Model file for the job. Use its own axes, mm. Face numbers are marked on the shaded views. A direction names the side the tool comes from. Coordinates: 2 decimals unless noted, no trailing zeros. Write each loop counter-clockwise with the first axis right and the second up, starting at its lowest first coordinate (ties: lowest second). Pieces come first, ordered by that corner, then holes. Notation, with made-up numbers: M -26.5,0 L 31.5,0 A3 ccw 31.5,5 Z; hole C 60.5,54 d5. An arc over 180 degrees is marked long. Put each result on its own line as item: value. Start each with the question number.
Q1. Drop flat-ended pins along their axis: pin 1 (5 mm diameter, centred on y = 238.5, z = 1.5, fed in from -X); pin 2 (6.5 mm diameter, centred on y = 335, z = 1.5, fed in from -X); pin 3 (5.5 mm diameter, centred on x = -24.5, y = 272, fed in from -Z); pin 4 (7 mm diameter, centred on y = 260, z = 141, fed in from -X). Give the stop position or say it passes through.
Q2. Which spindle directions (+Z, -Z, +X, -X, +Y, -Y) get a long thin tool onto all of the face, cutting with end or side? Do the marked faces 1 and 2. Say none if no direction does.
Q3. Cut at D-D (y = 188). Write the cut outline in (x, z).
Q4. Drill centre lines: line 1 along Y through (x, z) = (-2, 108); line 2 along Z through (x, y) = (-15, 181); line 3 along X through (y, z) = (195, 145.5). Where is each one in solid material? Low to high.
Q5. Cut at C-C (z = 108.38). Write the cut outline in (x, y), then the cut area to 3 significant figures.
Q6. Cut at A-A (z = 141). Write the cut outline in (x, y).
Q7. Cut at B-B (y = 230). Write the cut outline in (x, z).
Autodesk Inventor part; units mm, degrees
ref_plane "Work Plane1" through (-6, 230, 6) normal (0, -1, 0) x (1, 0, 0)
ref_plane "Work Plane2" through (-6, 190, 6) normal (0, -1, 0) x (1, 0, 0)
ref_plane "YZ Plane" through (0, 0, 0) normal (1, 0, 0) x (0, 1, 0)
sketch "Sketch1" plane through (0, 0, 0) normal (0, 0, 1) x (1, 0, 0)
  line L0 (0, 343) -> (-48.5, 343)
  line L1 (0, 343) -> (0, 113)
  line L2 (0, 113) -> (-48.5, 113)
  line L3 (-48.5, 113) -> (-48.5, 148)
  line L4 (-48.5, 148) -> (-32.5, 148)
  line L5 (-32.5, 148) -> (-32.5, 203)
  line L6 (-32.5, 203) -> (-13, 203)
  line L7 (-13, 203) -> (-13, 258)
  line L8 (-13, 258) -> (-32.5, 258)
  line L9 (-32.5, 258) -> (-32.5, 313)
  line L10 (-32.5, 313) -> (-48.5, 313)
  line L11 (-48.5, 313) -> (-48.5, 343)
  point P0 (0, 0)
  dimension "d0" = 230
  dimension "d1" = 13
  dimension "d2" = 30
  dimension "d3" = 55
  dimension "d4" = 55
  dimension "d5" = 55
  dimension "d6" = 16
extrude "Extrusion1" add sketch "Sketch1" along normal blind 6
fillet "Fillet1" radius 7 8 edges at (-32.5, 148, 3) (-32.5, 203, 3) (-13, 203, 3) (-13, 258, 3) (-32.5, 258, 3) (-32.5, 313, 3) (-48.5, 313, 3) (-48.5, 148, 3)
sketch "Sketch2" plane through (0, 0, 6) normal (0, 0, 1) x (1, 0, 0)
  line L0 (0, 113) -> (0, 343)
  line L1 (-6, 180) -> (0, 180)
  line L2 (0, 180) -> (0, 280)
  line L3 (0, 280) -> (-6, 280)
  line L4 (-6, 280) -> (-6, 180)
  line L5 (-15.5, 205) -> (-48.5, 205) construction
  line L6 (-48.5, 255) -> (-15.5, 255) construction
  line L7 (-15.5, 255) -> (-15.5, 205) construction
  line L8 (-15.5, 230) -> (0, 230) construction
  point P0 (0, 0)
  dimension "d10" = 100
  dimension "d11" = 6
extrude "Extrusion2" add sketch "Sketch2" along normal blind 241
sketch "Sketch3" plane through (-6, 180, 6) normal (-1, 0, 0) x (0, 0, 1)
  line L0 (241, 0) -> (241, 100)
  line L1 (235, 0) -> (235, 100)
  line L2 (241, 100) -> (241, 0)
  line L3 (241, 100) -> (241, 0)
  line L4 (241, 0) -> (241, -10)
  line L5 (241, -10) -> (235, -10)
  line L6 (235, -10) -> (235, 0)
  line L7 (235, 100) -> (235, 110)
  line L8 (235, 110) -> (241, 110)
  line L9 (0, 100) -> (241, 100) construction
  line L10 (241, 110) -> (241, 100)
  point P0 (-6, -180)
  dimension "d14" = 6
  dimension "d17" = 10
  dimension "d18" = 10
extrude "Extrusion3" add sketch "Sketch3" along normal blind 85
sketch "Sketch4" plane through (0, 0, 247) normal (0, 0, 1) x (1, 0, 0)
  line L0 (-37.6569, 174.8457) -> (-87.1543, 224.3431) construction
  line L1 (-87.1543, 235.6569) -> (-37.6569, 285.1543) construction
  line L2 (-40.4853, 172.0172) -> (-89.9828, 221.5147)
  line L3 (-91, 237.468) -> (-40.4853, 287.9828)
  line L4 (-89.9828, 221.5147) -> (-91, 222.532)
  line L5 (-91, 170) -> (-91, 290)
  line L6 (-89.9828, 238.4853) -> (-91, 237.468)
  line L7 (-40.4853, 287.9828) -> (-38.468, 290)
  line L8 (-6, 290) -> (-91, 290)
  line L9 (-40.4853, 172.0172) -> (-38.468, 170)
  line L10 (-6, 170) -> (-91, 170)
  line L11 (-38.468, 170) -> (-91, 170)
  line L12 (-6, 170) -> (-91, 170)
  line L13 (-91, 170) -> (-91, 222.532)
  line L14 (-91, 237.468) -> (-91, 290)
  line L15 (23.1543, 224.3431) -> (-26.3431, 174.8457) construction
  line L16 (-26.3431, 285.1543) -> (23.1543, 235.6569) construction
  line L17 (-18.7487, 292.7487) -> (30.7487, 243.2513) construction
  line L18 (30.7487, 216.7487) -> (-18.7487, 167.2513) construction
  line L19 (-6, 180) -> (0, 180)
  line L20 (-6, 170) -> (-6, 180)
  line L21 (-6, 180) -> (-6, 170)
  line L22 (-6, 170) -> (-16, 170)
  line L23 (-6, 180) -> (-16, 170)
  line L24 (-6, 280) -> (-6, 290)
  line L25 (-6, 280) -> (-6, 290)
  line L26 (-6, 290) -> (-16, 290)
  line L27 (-6, 280) -> (-16, 290)
  line L28 (-38.468, 290) -> (-91, 290)
  point P0 (0, 0)
  dimension "d19" = 4
  dimension "d20" = 4
extrude "Extrusion4" cut sketch "Sketch4" against normal blind 7
sketch "Sketch5" plane through (0, 113, 0) normal (1, 0, 0) x (0, 0, -1)
  line L0 (-241, 97) -> (-247, 97)
  line L1 (-247, 97) -> (-247, 137)
  line L2 (-247, 137) -> (-241, 137)
  line L3 (-241, 137) -> (-241, 97)
  line L4 (-247, 67) -> (-247, 167)
  point P0 (0, -113)
  point P1 (-247, 117)
  dimension "d25" = 6
  dimension "d26" = 40
extrude "Extrusion5" add sketch "Sketch5" along normal blind 26
chamfer "Chamfer1" distance 13 angle 45 4 edges at (0, 210, 244) (26, 210, 244) (26, 250, 244) (0, 250, 244)
sketch "Sketch6" plane through (0, 0, 247) normal (0, 0, 1) x (1, 0, 0)
  circle A0 centre (-32, 180.7854) radius 3.25
  circle A1 centre (-81.2146, 230) radius 3.25
  circle A2 centre (-32, 279.2146) radius 3.25
  circle A3 centre (17.2146, 230) radius 3.25
  circle A4 centre (-32, 230) radius 30 construction
  circle A5 centre (-32, 230) radius 30.5
  point P0 (0, 0)
  dimension "d33" = 0.5
extrude "Extrusion6" cut sketch "Sketch6" against normal blind 7
ref_plane "Work Plane1" through (-6, 230, 6) normal (0, -1, 0) x (1, 0, 0)
ref_plane "Work Plane2" through (-6, 190, 6) normal (0, -1, 0) x (1, 0, 0)
sketch "Sketch8" plane through (-6, 230, 6) normal (0, -1, 0) x (1, 0, 0)
  point P0 (6, -6)
sketch "Sketch11" plane through (-6, 230, 6) normal (0, -1, 0) x (1, 0, 0)
  point P0 (6, -6)
sketch "Sketch13" plane through (0, 0, 0) normal (0, 0, -1) x (-1, 0, 0)
  line L0 (0, 233) -> (0, 227)
  line L1 (0, 230) -> (0, 188)
  line L2 (0, 188) -> (24.5, 188)
  circle A0 centre (24.5, 188) radius 3.5
  line L3 (0, 230) -> (0, 156)
  line L4 (0, 113) -> (0, 180)
  line L5 (0, 156) -> (21.5, 156)
  circle A1 centre (21.5, 156) radius 4
  line L6 (0, 230) -> (0, 272)
  line L7 (0, 113) -> (0, 343)
  line L8 (0, 230) -> (0, 304)
  line L9 (0, 304) -> (21.5, 304)
  line L10 (0, 272) -> (24.5, 272)
  circle A2 centre (24.5, 272) radius 3.5
  circle A3 centre (21.5, 304) radius 4
  point P0 (0, 0)
  dimension "d56" = 42
  dimension "d57" = 24.5
  dimension "d58" = 7
  dimension "d59" = 74
  dimension "d60" = 21.5
  dimension "d61" = 8
  dimension "d62" = 42
  dimension "d63" = 74
  dimension "d64" = 7
  dimension "d65" = 8
sketch "Sketch15" plane through (-6, 280, 6) normal (-1, 0, 0) x (0, 0, 1)
  point P0 (-6, -280)
extrude "Extrusion19" cut sketch "Sketch13" against normal blind 16
sketch "Sketch23" plane through (0, 113, 0) normal (1, 0, 0) x (0, 0, -1)
  circle A0 centre (-108.38, 91) radius 4.5
  line L0 (-6, 67) -> (-247, 67)
  line L1 (-6, 0) -> (-6, 230)
  line L2 (0, 0) -> (0, 230) construction
  circle A1 centre (-108.38, 143) radius 4.5
  line L3 (-6, 167) -> (-6, 230)
  line L4 (-6, 167) -> (-247, 167)
  point P0 (0, -113)
  point P1 (-61, 67)
  point P2 (-6, 55)
  point P3 (-6, 179)
  point P4 (-61, 167)
  dimension "d87" = 9
  dimension "d88" = 24
  dimension "d89" = 102.38
  dimension "d90" = 9
  dimension "d91" = 102.38
  dimension "d92" = 24
extrude "Extrusion20" cut sketch "Sketch23" against normal through all
sketch "Sketch24" plane through (-6, 180, 6) normal (-1, 0, 0) x (0, 0, 1)
  circle A0 centre (135, 80) radius 4
  circle A1 centre (135, 20) radius 4
  line L0 (0, 0) -> (235, 0)
  line L1 (0, 100) -> (235, 100)
  line L2 (0, 71) -> (0, 30)
  point P0 (-6, -180)
  dimension "d95" = 8
  dimension "d96" = 8
  dimension "d97" = 20
  dimension "d98" = 20
  dimension "d99" = 135
extrude "Extrusion21" cut sketch "Sketch24" against normal blind 10
equation "\"d98\" = d97"
properties part number "X axis screw support" material "Steel"
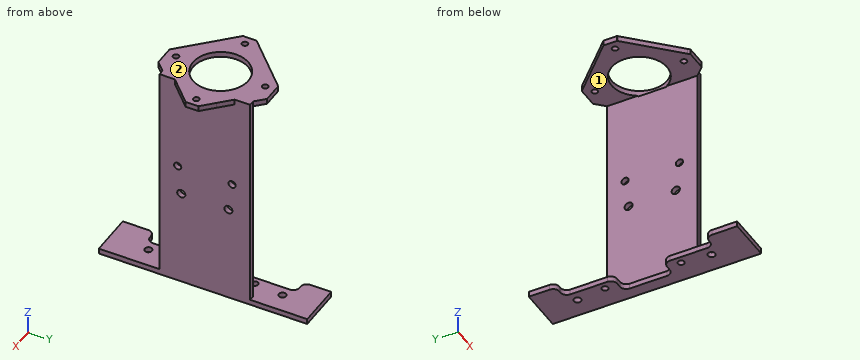
Computed values:
1. pin 1: x = -13
1. pin 2: x = -48.5
1. pin 3: z = 241
1. pin 4: through
2. face 1: -X, +Y, -Y
2. face 2: +Z, +X, -X, +Y, -Y
3. outline: M -56.47,241 L -6,241 L -6,6 L -21,6 L -21,0 L 0,0 L 0,247 L -56.47,247 Z; M -32.5,0 L -28,0 L -28,6 L -32.5,6 Z
4. line 1: 180 to 199.52, 208.48 to 251.52, 260.48 to 280
4. line 2: 0 to 6, 241 to 247
4. line 3: -6 to 0
5. outline: M -6,180 L 0,180 L 0,199.5 L -6,199.5 Z; M -6,208.5 L 0,208.5 L 0,251.5 L -6,251.5 Z; M -6,260.5 L 0,260.5 L 0,280 L -6,280 Z
5. area: 492 mm2
6. outline: M -6,180 L 0,180 L 0,196 L -6,196 Z; M -6,204 L 0,204 L 0,256 L -6,256 Z; M -6,264 L 0,264 L 0,280 L -6,280 Z
7. outline: M -91,241 L -84.46,241 L -84.46,247 L -91,247 Z; M -77.96,241 L -62.5,241 L -62.5,247 L -77.96,247 Z; M -13,0 L 0,0 L 0,241 L 13.96,241 L 13.96,247 L -1.5,247 L -1.5,240 L -6,240 L -6,6 L -13,6 Z; M 20.46,241 L 26,241 L 26,247 L 20.46,247 Z
